```python
from build123d import *

# Parameters (mm, degrees)
F0_R     = 67
F0_W     = 3.2
F0_H     = 5.2
F1_DEPTH = 5


with BuildPart() as f1:
    # F0 (on Top) → F1 (new body)
    with BuildSketch(Plane.XY):
        Circle(F0_R)
        with BuildLine():
            Line((-43.8061632072, -42.4502068907), (-27.7453339126, -37.5246361488))
            Line((-27.7453339126, -37.5246361488), (-27.7453339126, -54.3249155184))
            ThreePointArc((-27.7453339126, -54.3249155184), (-36.2650846031, -49.0493999834), (-43.8061632072, -42.4502068907))
        make_face(mode=Mode.SUBTRACT)
        with BuildLine():
            Line((-24.5453339126, -36.543253053), (-16.2077082994, -33.9862515417))
            Line((-16.2077082994, -33.9862515417), (-15.32809766, -36.8544016639))
            Line((-15.32809766, -36.8544016639), (-4.620337204, -33.5705219434))
            Line((-4.620337204, -33.5705219434), (-5.4999478434, -30.7023718213))
            Line((-5.4999478434, -30.7023718213), (12.0330121636, -25.3253247681))
            Line((12.0330121636, -25.3253247681), (21.7448194921, -56.9926558888))
            ThreePointArc((21.7448194921, -56.9926558888), (-1.5135076095, -60.9812208365), (-24.5453339126, -55.8437694208))
            Line((-24.5453339126, -55.8437694208), (-24.5453339126, -36.543253053))
        make_face(mode=Mode.SUBTRACT)
        with BuildLine():
            Line((-27.7453339126, -2.5714068584), (-27.7453339126, -34.1775310144))
            Line((-27.7453339126, -34.1775310144), (-46.1961790611, -39.8360771181))
            ThreePointArc((-46.1961790611, -39.8360771181), (-55.6535662863, -24.9735972503), (-60.469385046, -8.0282919824))
            Line((-60.469385046, -8.0282919824), (-59.8046514096, -7.9174446097))
            Line((-59.8046514096, -7.9174446097), (-27.7453339126, -2.5714068584))
        make_face(mode=Mode.SUBTRACT)
        Polygon((-13.3395581772, -33.1066409023), (-14.2778095259, -30.0472807721), (-9.3063493142, -28.5226223304), (-8.3680979656, -31.5819824607), align=None, mode=Mode.SUBTRACT)
        Polygon((-18.0255702875, -28.0587412893), (-17.1459596481, -30.9268914115), (-24.5453339126, -33.1961479186), (-24.5453339126, -2.0377922297), (3.4589808569, 2.6320552794), (11.0947608149, -22.2659646378), (-6.4381991921, -27.643011691), (-7.3178098315, -24.7748615689), align=None, mode=Mode.SUBTRACT)
        with BuildLine():
            Line((15.0923722939, -24.3870734194), (29.0776945802, -20.098023769))
            Line((29.0776945802, -20.098023769), (35.0708025243, -49.9103076559))
            ThreePointArc((35.0708025243, -49.9103076559), (30.0367604433, -53.0923066185), (24.7164230966, -55.7682564665))
            Line((24.7164230966, -55.7682564665), (15.0923722939, -24.3870734194))
        make_face(mode=Mode.SUBTRACT)
        with BuildLine():
            Line((37.9086808974, -47.790500234), (32.2192885129, -19.4890275267))
            Line((32.2192885129, -19.4890275267), (35.16044758, -18.8977717934))
            Line((35.16044758, -18.8977717934), (35.0344853908, -18.2711819544))
            Line((35.0344853908, -18.2711819544), (60.0733303031, -10.5922134746))
            ThreePointArc((60.0733303031, -10.5922134746), (52.402736228, -31.2242411568), (37.9086808974, -47.790500234))
        make_face(mode=Mode.SUBTRACT)
        Polygon((31.6280327797, -16.5478684596), (28.4907964414, -17.1785412418), (27.4659531704, -12.0805321921), (30.6031895087, -11.44985941), align=None, mode=Mode.SUBTRACT)
        Polygon((23.8255728418, 6.0282775984), (26.8746974372, -9.1393731251), (23.9335383701, -9.7306288583), (25.5615882832, -17.8292459105), (14.1541209452, -21.3277132891), (6.6432408292, 3.1630451865), align=None, mode=Mode.SUBTRACT)
        with BuildLine():
            Line((60.5868434596, -7.0876229867), (34.400697228, -15.1184483792))
            Line((34.400697228, -15.1184483792), (32.9530928425, -7.9174446097))
            Line((32.9530928425, -7.9174446097), (30.0119337754, -8.5087003429))
            Line((30.0119337754, -8.5087003429), (26.9837234891, 6.5549136562))
            Line((26.9837234891, 6.5549136562), (59.802483499, 12.0275919182))
            ThreePointArc((59.802483499, 12.0275919182), (60.9487109921, 2.5009255083), (60.5868434596, -7.0876229867))
        make_face(mode=Mode.SUBTRACT)
        with BuildLine():
            Line((-30.7453339126, 14.2669440508), (-27.7453339126, 14.2669440508))
            Line((-27.7453339126, 14.2669440508), (-27.7453339126, 0.6727794143))
            Line((-27.7453339126, 0.6727794143), (-60.8076429886, -4.8405117679))
            ThreePointArc((-60.8076429886, -4.8405117679), (-60.5773112158, 7.1686376578), (-57.9982415713, 18.899840598))
            Line((-57.9982415713, 18.899840598), (-30.7453339126, 21.6120113579))
            Line((-30.7453339126, 21.6120113579), (-30.7453339126, 14.2669440508))
        make_face(mode=Mode.SUBTRACT)
        Polygon((-24.5453339126, 1.206394043), (-24.5453339126, 14.2669440508), (-21.5453339126, 14.2669440508), (-21.5453339126, 22.5275823238), (-3.2024586813, 24.3530392797), (2.5124526937, 5.7184036538), align=None, mode=Mode.SUBTRACT)
        Polygon((0.0455163714, 24.6762731554), (11.7609695409, 25.842178457), (12.0580577422, 22.8569249334), (20.278090913, 23.6749709889), (23.1945533758, 9.1672384904), (5.6967126659, 6.249393561), align=None, mode=Mode.SUBTRACT)
        with Locations((-26.1453339126, 19.8669440508)):
            Rectangle(F0_W, F0_H, mode=Mode.SUBTRACT)
        with BuildLine():
            Line((-27.7453339126, 54.3249155184), (-27.7453339126, 25.4669440508))
            Line((-27.7453339126, 25.4669440508), (-30.7453339126, 25.4669440508))
            Line((-30.7453339126, 25.4669440508), (-30.7453339126, 24.8278186332))
            Line((-30.7453339126, 24.8278186332), (-56.8033838043, 22.2345584255))
            ThreePointArc((-56.8033838043, 22.2345584255), (-45.2169124497, 40.9442404804), (-27.7453339126, 54.3249155184))
        make_face(mode=Mode.SUBTRACT)
        with BuildLine():
            Line((-4.1594807198, 27.4736050776), (-24.5453339126, 25.4448338493))
            Line((-24.5453339126, 25.4448338493), (-24.5453339126, 55.8437694208))
            ThreePointArc((-24.5453339126, 55.8437694208), (-19.3268992288, 57.8573328646), (-13.9459622608, 59.384426718))
            Line((-13.9459622608, 59.384426718), (-4.1594807198, 27.4736050776))
        make_face(mode=Mode.SUBTRACT)
        with BuildLine():
            Line((11.1469872581, 32.011702406), (11.4440754595, 29.0264488823))
            Line((11.4440754595, 29.0264488823), (-0.9115056672, 27.7968389533))
            Line((-0.9115056672, 27.7968389533), (-10.7988456048, 60.036529993))
            ThreePointArc((-10.7988456048, 60.036529993), (1.1523404732, 60.9891146963), (13.0590128663, 59.5857548661))
            Line((13.0590128663, 59.5857548661), (18.4559499448, 32.7390800176))
            Line((18.4559499448, 32.7390800176), (11.1469872581, 32.011702406))
        make_face(mode=Mode.SUBTRACT)
        Polygon((19.6037684242, 29.838489966), (19.9206625056, 26.6542195407), (14.7462230646, 26.1392666584), (14.4293289831, 29.3235370836), align=None, mode=Mode.SUBTRACT)
        with BuildLine():
            Line((22.8839145104, 26.9491181821), (22.9059160293, 26.951307742))
            Line((22.9059160293, 26.951307742), (53.1358049871, 29.9597434631))
            ThreePointArc((53.1358049871, 29.9597434631), (56.5982407155, 22.7516845071), (59.0880479964, 15.1526428049))
            Line((59.0880479964, 15.1526428049), (26.3527040231, 9.6938745483))
            Line((26.3527040231, 9.6938745483), (22.8839145104, 26.9491181821))
        make_face(mode=Mode.SUBTRACT)
        with BuildLine():
            ThreePointArc((16.4956071696, 58.7272930085), (36.2609976032, 49.0524214776), (51.3071590572, 32.9935664862))
            Line((51.3071590572, 32.9935664862), (22.5890219478, 30.1355781673))
            Line((22.5890219478, 30.1355781673), (22.2919337465, 33.120831691))
            Line((22.2919337465, 33.120831691), (21.6559499448, 33.0575394841))
            Line((21.6559499448, 33.0575394841), (16.4956071696, 58.7272930085))
        make_face(mode=Mode.SUBTRACT)
    extrude(amount=F1_DEPTH)


solid = f1.part
```
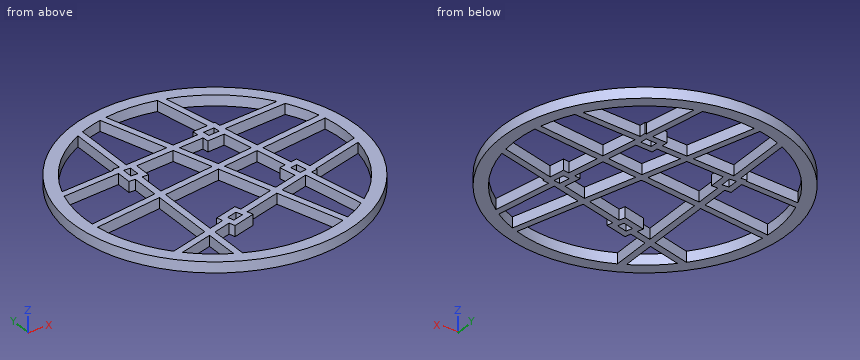
For this review, take the finished solid that the model builds, in its own axes (mm). Give positions to 0.01 mm unless a question says otherwise; leave off trailing zeros. Order: outer loops, then holes, each group sorted by start corner. A loop starts at its lowest first (then second) coordinate and runs counter-clockwise, first axis right, second up.
1) Wall thickness on line 1 (Y direction, x = -29, z = 1.1); line 2 (Y direction, x = -16.5, z = 1.8); line 3 (X direction, y = 35.5, z = 0.8): over which ranges is each line inside the solid? List them lowest first.
2) Take a section at C-C (z = 3.15). State how many separate pieces and enclosed holes the cut face has, then the cut area to 3 significant figures.
3) Take a section at B-B (y = 44.5). Give the boundary of the cut face in (x, z).
4) Insertion check: pin 1 (2.5 mm diameter, centred on y = -44.5, z = 3.5, fed in from -X); pin 2 (2.5 mm diameter, centred on y = -43, z = 3.5, fed in from +X); pin 3 (1.5 mm diameter, centred on y = 7.5, z = 2.5, fed in from -X); pin 4 (8 mm diameter, centred on x = 11, y = 16, fed in from -Z). Each pin has a flat end and moves straight along its axis. Give the tip position at first contact, or say it passes through.
5) Take a section at A-A (x = 56). Give the boundary of the cut face in (y, z), then the cut area to 3 significant figures.
Derived:
1. line 1: y = -60.4 to -53.67, -37.91 to -34.56, -2.78 to 0.46, 14.27 to 25.47, 53.67 to 60.4
1. line 2: y = -64.94 to -58.73, -34.08 to -27.59, -0.7 to 2.55, 23.03 to 26.25, 58.73 to 64.94
1. line 3: x = -56.82 to -49.61, -27.75 to -24.55, -6.62 to -3.27, 17.9 to 21.16, 49.61 to 56.82
2. separate pieces: 1
2. enclosed holes: 20
2. area: 4,650 mm2
3. outline: (-50.09, 0) - (-41.72, 0) - (-41.72, 5) - (-50.09, 5) - close; (-27.75, 0) - (-24.55, 0) - (-24.55, 5) - (-27.75, 5) - close; (-9.38, 0) - (-6.03, 0) - (-6.03, 5) - (-9.38, 5) - close; (16.09, 0) - (19.36, 0) - (19.36, 5) - (16.09, 5) - close; (41.72, 0) - (50.09, 0) - (50.09, 5) - (41.72, 5) - close
4. pin 1: stops at x = -51.17
4. pin 2: stops at x = 52.4
4. pin 3: stops at x = -66.66
4. pin 4: passes through
5. outline: (-36.78, 0) - (-24.19, 0) - (-24.19, 5) - (-36.78, 5) - close; (-11.84, 0) - (-8.49, 0) - (-8.49, 5) - (-11.84, 5) - close; (11.39, 0) - (14.64, 0) - (14.64, 5) - (11.39, 5) - close; (24.19, 0) - (36.78, 0) - (36.78, 5) - (24.19, 5) - close
5. area: 159 mm2
